Input: part model. Units: mm. Frame: model coordinates. Coordinates: 2 decimals unless noted, no trailing zeros. Write each loop counter-clockwise with the first axis right and the second up, starting at its lowest first coordinate (ties: lowest second). Pieces come first, ordered by that corner, then holes. Notation, with made-up numbers: (34.5, -30.75) -> (71.5, -30.75) arc R20 ccw to (71.5, 1.25) -> close; hole circle Ø9 at (-11, -34.5). An arc over 180 degrees is marked (long way). One line per question, with ' | ' between items. Start each with the question number.
```python
from build123d import *

# Parameters (mm, degrees)
SKETCH_W     = 59
SKETCH_H     = 20
SKETCH_R     = 1.5
SKETCH_R_2   = 1.6
SKETCH_W_2   = 13
SKETCH_H_2   = 8
PAD_DEPTH    = 3
SKETCH002_W  = 25
SKETCH002_H  = 8
POCKET_DEPTH = 1.7


with BuildPart() as part:
    # Sketch → Pad (new body)
    with BuildSketch(Plane.XY):
        Rectangle(SKETCH_W, SKETCH_H)
        with Locations((-22.5, 0)):
            Circle(SKETCH_R, mode=Mode.SUBTRACT)
        with Locations((-8.5, 0)):
            Circle(SKETCH_R_2, mode=Mode.SUBTRACT)
        with Locations((8.5, 0)):
            Circle(SKETCH_R_2, mode=Mode.SUBTRACT)
        with Locations((22.5, 0)):
            Circle(SKETCH_R, mode=Mode.SUBTRACT)
        Rectangle(SKETCH_W_2, SKETCH_H_2, mode=Mode.SUBTRACT)
    extrude(amount=PAD_DEPTH)

    # Sketch002 (on Face14 of Pad) → Pocket (cut)
    with BuildSketch(Plane.XY.offset(3)):
        Rectangle(SKETCH002_W, SKETCH002_H)
    extrude(amount=-POCKET_DEPTH, mode=Mode.SUBTRACT)


solid = part.part
```
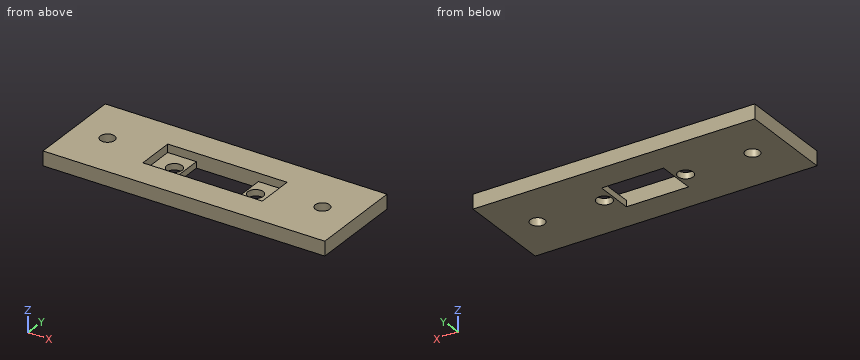
1) Section D-D, the plane y = -3.25. Return loops of the section in (x, z), then the cut area to 3 significant figures.
2) Section A-A, the plane y = 0. Return loops of the section in (x, z), then the cut area to 3 significant figures.
3) Section B-B, the plane x = -1. Return loops of the section in (y, z), then the cut area to 3 significant figures.
4) First-contact query: P1, Ø1.5, axis at x = 4, y = -2.5, coming from the +Z side; P2, Ø1.8, axis at x = -10, y = -1.5, coming from the +Z side. Flat tips, straight axial feed; report the tip coordinate or a pass-through.
5) Ray query, line 1 (Y direction, x = 10, z = 2.05); line 2 (X direction, y = 1.25, z = 2.6); line 3 (Y direction, x = -8.5, z = 0.65). Return the intervals inside material, ascending.
6) Section C-C, the plane z = 2. Return loops of the section in (x, y), then the cut area to 3 significant figures.
Answer block:
1) outline: (-29.5, 0) -> (-6.5, 0) -> (-6.5, 1.3) -> (-12.5, 1.3) -> (-12.5, 3) -> (-29.5, 3) -> close; (6.5, 0) -> (29.5, 0) -> (29.5, 3) -> (12.5, 3) -> (12.5, 1.3) -> (6.5, 1.3) -> close | area: 118 mm2
2) outline: (-29.5, 0) -> (-24, 0) -> (-24, 3) -> (-29.5, 3) -> close; (-21, 0) -> (-10.1, 0) -> (-10.1, 1.3) -> (-12.5, 1.3) -> (-12.5, 3) -> (-21, 3) -> close; (-6.9, 0) -> (-6.5, 0) -> (-6.5, 1.3) -> (-6.9, 1.3) -> close; (6.5, 0) -> (6.9, 0) -> (6.9, 1.3) -> (6.5, 1.3) -> close; (10.1, 0) -> (21, 0) -> (21, 3) -> (12.5, 3) -> (12.5, 1.3) -> (10.1, 1.3) -> close; (24, 0) -> (29.5, 0) -> (29.5, 3) -> (24, 3) -> close | area: 91.3 mm2
3) outline: (-10, 0) -> (-4, 0) -> (-4, 3) -> (-10, 3) -> close; (4, 0) -> (10, 0) -> (10, 3) -> (4, 3) -> close | area: 36.0 mm2
4) P1: passes through | P2: stops at z = 1.3
5) line 1: y = -10 to -4, 4 to 10 | line 2: x = -29.5 to -23.33, -21.67 to -12.5, 12.5 to 21.67, 23.33 to 29.5 | line 3: y = -10 to -1.6, 1.6 to 10
6) outline: (-29.5, -10) -> (29.5, -10) -> (29.5, 10) -> (-29.5, 10) -> close; hole circle Ø3 at (-22.5, 0); hole (-12.5, -4) -> (12.5, -4) -> (12.5, 4) -> (-12.5, 4) -> close; hole circle Ø3 at (22.5, 0) | area: 966 mm2
